Geometry check sheet. Reference: the model listing, model coordinates, mm. A direction names the side the tool comes from. Round coordinates to 2 decimals unless told otherwise and drop trailing zeros. Loops run counter-clockwise (first coordinate to the right, second up) from the corner with the lowest first, then second, coordinate; pieces in that order, holes last.
```python
from build123d import *

# Parameters (mm, degrees)
SKETCH1_W                = 20
SKETCH1_H                = 115
BOSS_EXTRUDE1_DEPTH      = 5
CHAMFER1_SIZE            = 1
CHAMFER2_SIZE            = 1
M3_CLEARANCE_HOLE6_D     = 3.6
M3_CLEARANCE_HOLE6_DEPTH = 5
SKETCH19_W               = 10.75
SKETCH19_H               = 7
CUT_EXTRUDE3_DEPTH       = 6
SKETCH20_R               = 3.375
CUT_EXTRUDE4_DEPTH       = 10


with BuildPart() as part:
    # Sketch1 → Boss-Extrude1 (new body)
    with BuildSketch(Plane(origin=(0, 0, 0), x_dir=(1, 0, 0), z_dir=(0, 1, 0))):
        with Locations((10, 57.5)):
            Rectangle(SKETCH1_W, SKETCH1_H)
    extrude(amount=BOSS_EXTRUDE1_DEPTH)

    # Chamfer1
    chamfer1_edges = [part.edges().sort_by_distance(p)[0] for p in [
        (20, 5, -57.5),
        (0, 5, -57.5),
        (20, 0, -57.5),
        (0, 0, -57.5),
        (0, 2.5, -115),
        (20, 2.5, -115),
        (20, 2.5, 0),
        (0, 2.5, 0),
    ]]
    chamfer(chamfer1_edges, length=CHAMFER1_SIZE)

    # Chamfer2
    chamfer2_edges = [part.edges().sort_by_distance(p)[0] for p in [
        (10, 5, -115),
        (10, 0, -115),
    ]]
    chamfer(chamfer2_edges, length=CHAMFER2_SIZE)

    # M3 Clearance Hole6
    with Locations(Plane(origin=(0, 0, 0), x_dir=(-1, 0, 0), z_dir=(0, -1, 0))):
        with Locations((-10, 109), (-10, 99)):
            Hole(M3_CLEARANCE_HOLE6_D / 2, depth=M3_CLEARANCE_HOLE6_DEPTH)

    # Sketch19 → Cut-Extrude3 (cut, through all)
    with BuildSketch(Plane(origin=(0, 0, 0), x_dir=(1, 0, 0), z_dir=(0, 1, 0))):
        with Locations((10, 20.704322589)):
            Rectangle(SKETCH19_W, SKETCH19_H)
    cut_extrude3 = extrude(amount=CUT_EXTRUDE3_DEPTH, mode=Mode.SUBTRACT)

    # Mirror1: Cut-Extrude3 across plane
    add(cut_extrude3.mirror(Plane.XY.offset(-28.391822589)), mode=Mode.SUBTRACT)

    # Sketch20 → Cut-Extrude4 (cut)
    with BuildSketch(Plane(origin=(0, 5, 0), x_dir=(1, 0, 0), z_dir=(0, 1, 0))):
        with Locations((10, 50)):
            Circle(SKETCH20_R)
    extrude(amount=-CUT_EXTRUDE4_DEPTH, mode=Mode.SUBTRACT)


solid = part.part
```
1) Sectioned sample at A-A, the plane z = -109. Record the cut outline in (x, y).
Report:
outline: (0, 1) - (1, 0) - (8.2, 0) - (8.2, 5) - (1, 5) - (0, 4) - close; (11.8, 0) - (19, 0) - (20, 1) - (20, 4) - (19, 5) - (11.8, 5) - close
2) Sectioned sample at C-C, the plane z = -31. Record the cut outline in (x, y), then the cut area to 3 significant figures.
Report:
outline: (0, 1) - (1, 0) - (19, 0) - (20, 1) - (20, 4) - (19, 5) - (1, 5) - (0, 4) - close
area: 98.0 mm2
3) Access from +Z, -Z, +X, -X, +Y, -Y to the whole of each face (thin tool, end or side, straight path). Record for faces 1 (the face through (10, 5, -58)), 2 (the face through (4.625, 2, -36)).
Report:
face 1: +Z, -Z, +X, -X, +Y
face 2: +Y, -Y
4) Sectioned sample at B-B, the plane z = -50. Record the cut outline in (x, y) (3 decimals).
Report:
outline: (0, 1) - (1, 0) - (6.625, 0) - (6.625, 5) - (1, 5) - (0, 4) - close; (13.375, 0) - (19, 0) - (20, 1) - (20, 4) - (19, 5) - (13.375, 5) - close
5) Scan lines: line 1 along Z through (x, y) = (6.5, 1.4); line 2 along Z through (x, y) = (9.75, 2.6); line 3 along X through (y, z) = (2.85, -50) (3 decimals). Record each from-to range of solid material in increasing order.
Report:
line 1: z = -115 to -39.58, -32.58 to -24.2, -17.2 to 0
line 2: z = -115 to -110.78, -107.22 to -100.78, -97.22 to -53.37, -46.63 to -39.58, -32.58 to -24.2, -17.2 to 0
line 3: x = 0 to 6.625, 13.375 to 20
6) Mould release check, pull along X, two halves, no side actions. Record for faces 3 (the face through (20, 2, -57)), 4 (the face through (10, 0, -58)), 5 (the face through (0, 2, -57)), 6 (the face through (10.831, 2.535, -107.403)): +X half, -X half, draft (parallel to the pull), parting line (faces both ways), or undercut.
Report:
face 3: +X half
face 4: draft
face 5: -X half
face 6: undercut
7) Gauge pin test, flat end, axial feed: pin 1 (3 mm diameter, centred on x = 10, z = -99, fed in from +Y). Record the tip position at first contact, or that the pin passes through.
Report:
pin 1: passes through
